Input: part model. Units: mm. Frame: model coordinates. A direction names the side the tool comes from. Coordinates: 2 decimals unless noted, no trailing zeros. Order: outer loops, then holes, each group sorted by start corner. A loop starts at its lowest first (then second) coordinate and runs counter-clockwise, first axis right, second up. Notation, with made-up numbers: (64.25, 52) - (110.25, 52) arc R22 cw to (110.25, 65) - close; hole circle Ø10 at (-30.5, 34.25). An arc over 180 degrees is marked (long way). Answer as CSV lines item,"result". Start each with the question number.
Item 1: Section A-A (x = 38.1). Output: boundary loops of the cut face in (y, z).
Item 2: Section C-C (y = 0). Output: boundary loops of the cut face in (x, z).
Item 3: Section D-D (x = 0). Output: boundary loops of the cut face in (y, z).
Item 4: Draft query along Y for faces 4 (the flat face through (-1, -25.4, 11)), 5 (the cylindrical face through (-34.686, 18.054, 12.878)), 6 (the flat face through (50.8, 0, 11)). Return one class per face: +Y half, -Y half, draft (parallel to the pull), parting line (faces both ways), or undercut.
Item 5: Access query for faces 1 (the cylindrical face through (1.38, 6.2, 57.24)), 2 (the cylindrical face through (2.75, 12.4, 69.9)), 3 (the cylindrical face through (31.756, -12.421, 12.878)). Directions: +Z, -Z, +X, -X, +Y, -Y. A direction counts if a zero-diameter tool reaches every point of the face in a straight line with its end or side. Return the directions, or none.
Item 6: Material intervals for line 1 along Y through (x, z) = (38.1, 13); line 2 along Y through (x, z) = (35, 25); line 3 along Z through (x, y) = (6.5, -3), sorted ascending.
Item 7: Section B-B (z = 16.5). Output: boundary loops of the cut face in (x, y), and give its area (3 significant figures).
Item 8: First-contact query: pin 1 (12 mm diameter, centred on x = 2.5, y = 20, fed in from -Z); pin 2 (10 mm diameter, centred on x = -5, z = 49, fed in from -Y); pin 3 (10 mm diameter, centred on y = 12.5, z = 44, fed in from +X); pin 4 (12 mm diameter, centred on y = -10.5, z = 39, fed in from +X). Flat tips, straight axial feed; report the tip coordinate or a pass-through.
from build123d import *

# Parameters (mm, degrees)
F0_W     = 101.6
F0_H     = 50.8
F1_DEPTH = 25.4
F2_R     = 6.35
F3_DEPTH = 25.401
F4_W     = 12.7
F4_H     = 50.8
F6_W     = 18.9611997128
F6_H     = 12.7
F8_R     = 2.54
F9_SIZE  = 2.54


with BuildPart() as f1:
    # F0 (on Top) → F1 (new body)
    with BuildSketch(Plane.XY):
        Rectangle(F0_W, F0_H)
    extrude(amount=F1_DEPTH)

    # F2 (on face) → F3 (cut, through all)
    with BuildSketch(Plane.XY.offset(25.4)):
        with Locations((38.1, -12.7)):
            Circle(F2_R)
        with Locations((38.1, 12.7)):
            Circle(F2_R)
        with Locations((-38.1, 12.7)):
            Circle(F2_R)
        with Locations((-38.1, -12.7)):
            Circle(F2_R)
    extrude(amount=-F3_DEPTH, mode=Mode.SUBTRACT)

    # F4 (on Front) → F5 (revolve)
    with BuildSketch(Plane.XZ):
        with Locations((-6.35, 50.8)):
            Rectangle(F4_W, F4_H)
    revolve(axis=Axis((0, 0, 50.8), (0, 0, 1)))

    # F6 (on Front) → F7 (revolve, cut)
    with BuildSketch(Plane.XZ):
        with Locations((-15.8305998564, 57.15)):
            Rectangle(F6_W, F6_H)
    revolve(axis=Axis((0, 0, 46.6448366642), (0, 0, 1)), mode=Mode.SUBTRACT)

    # F8
    f8_edges = [f1.edges().sort_by_distance(p)[0] for p in [
        (12.7, 0, 50.8),
        (12.7, 0, 76.2),
        (12.7, 0, 25.4),
        (12.7, 0, 63.5),
    ]]
    fillet(f8_edges, radius=F8_R)

    # F9
    f9_edges = [f1.edges().sort_by_distance(p)[0] for p in [
        (0, 25.4, 25.4),
        (50.8, 0, 25.4),
        (0, -25.4, 25.4),
        (-50.8, 0, 25.4),
    ]]
    chamfer(f9_edges, length=F9_SIZE)


solid = f1.part
Determined:
1,outline,"(-25.4, 0) - (-19.05, 0) - (-19.05, 25.4) - (-22.86, 25.4) - (-25.4, 22.86) - close; (-6.35, 0) - (6.35, 0) - (6.35, 25.4) - (-6.35, 25.4) - close; (19.05, 0) - (25.4, 0) - (25.4, 22.86) - (22.86, 25.4) - (19.05, 25.4) - close"
2,outline,"(-50.8, 0) - (50.8, 0) - (50.8, 22.86) - (48.26, 25.4) - (15.24, 25.4) arc R2.54 cw to (12.7, 27.94) - (12.7, 48.26) arc R2.54 ccw to (10.16, 50.8) - (6.35, 50.8) - (6.35, 63.5) - (10.16, 63.5) arc R2.54 ccw to (12.7, 66.04) - (12.7, 73.66) arc R2.54 ccw to (10.16, 76.2) - (-10.16, 76.2) arc R2.54 ccw to (-12.7, 73.66) - (-12.7, 66.04) arc R2.54 ccw to (-10.16, 63.5) - (-6.35, 63.5) - (-6.35, 50.8) - (-10.16, 50.8) arc R2.54 ccw to (-12.7, 48.26) - (-12.7, 27.94) arc R2.54 cw to (-15.24, 25.4) - (-48.26, 25.4) - (-50.8, 22.86) - close"
3,outline,"(-25.4, 0) - (25.4, 0) - (25.4, 22.86) - (22.86, 25.4) - (15.24, 25.4) arc R2.54 cw to (12.7, 27.94) - (12.7, 48.26) arc R2.54 ccw to (10.16, 50.8) - (6.35, 50.8) - (6.35, 63.5) - (10.16, 63.5) arc R2.54 ccw to (12.7, 66.04) - (12.7, 73.66) arc R2.54 ccw to (10.16, 76.2) - (-10.16, 76.2) arc R2.54 ccw to (-12.7, 73.66) - (-12.7, 66.04) arc R2.54 ccw to (-10.16, 63.5) - (-6.35, 63.5) - (-6.35, 50.8) - (-10.16, 50.8) arc R2.54 ccw to (-12.7, 48.26) - (-12.7, 27.94) arc R2.54 cw to (-15.24, 25.4) - (-22.86, 25.4) - (-25.4, 22.86) - close"
4,face 4,"-Y half"
4,face 5,"undercut"
4,face 6,"draft"
5,face 1,"none"
5,face 2,"+Z"
5,face 3,"+Z, -Z"
6,line 1,"y = -25.4 to -19.05, -6.35 to 6.35, 19.05 to 25.4"
6,line 2,"y = -23.26 to -18.24, -7.16 to 7.16, 18.24 to 23.26"
6,line 3,"z = 0 to 50.8, 63.5 to 76.2"
7,outline,"(-50.8, -25.4) - (50.8, -25.4) - (50.8, 25.4) - (-50.8, 25.4) - close; hole circle Ø12.7 at (-38.1, -12.7); hole circle Ø12.7 at (-38.1, 12.7); hole circle Ø12.7 at (38.1, -12.7); hole circle Ø12.7 at (38.1, 12.7)"
7,area,"4,650 mm^2"
8,pin 1,"stops at z = 0"
8,pin 2,"stops at y = -12.7"
8,pin 3,"stops at x = 10.25"
8,pin 4,"stops at x = 11.88"
